Verification items for the finished model (mm, model axes). A direction names the side the tool comes from. Round coordinates to 2 decimals unless told otherwise and drop trailing zeros. Write each loop counter-clockwise with the first axis right and the second up, starting at its lowest first coordinate (ties: lowest second). Pieces come first, ordered by that corner, then holes. Notation, with made-up numbers: M 21.5,48 L 60.5,48 A11 ccw 60.5,64 Z; hole C 20,47.5 d3. An arc over 180 degrees is marked long. One line per question, with ' | ' between items.
Autodesk Inventor part; units mm, degrees
ref_plane "YZ Plane" through (0, 0, 0) normal (1, 0, 0) x (0, 1, 0)
ref_plane "XZ Plane" through (0, 0, 0) normal (0, 1, 0) x (-1, 0, 0)
ref_plane "XY Plane" through (0, 0, 0) normal (0, 0, 1) x (1, 0, 0)
sketch "Sketch1" plane through (0, 0, 0) normal (0, 1, 0) x (-1, 0, 0)
  line L0 (-2.45, -18) -> (2.45, -18)
  line L1 (2.45, -18) -> (2.45, 18)
  line L2 (2.45, 18) -> (-2.45, 18)
  line L3 (-2.45, 18) -> (-2.45, -18)
  line L4 (-2.45, -18) -> (2.45, 18) construction
  line L5 (2.45, -18) -> (-2.45, 18) construction
  point P0 (0, 0)
  dimension "d0" = 36
  dimension "d1" = 4.9
extrude "Extrusion1" add sketch "Sketch1" along normal blind 12
sketch "Sketch2" plane through (2.45, 0, 18) normal (1, 0, 0) x (0, 0, -1)
  circle A0 centre (26, 7) radius 2.5
  line L0 (36, 0) -> (36, 12)
  line L1 (0, 12) -> (36, 12)
  point P0 (18, 0)
  dimension "d4" = 5
  dimension "d5" = 10
  dimension "d18" = 5
fillet "Fillet1" radius 5 2 edges at (0, 12, -18) (0, 0, -18)
sketch "Sketch3" plane through (2.45, 0, 18) normal (1, 0, 0) x (0, 0, -1)
  line L0 (0, 0) -> (0, -15)
  arc A0 (36, 7) -> (31, 12) centre (31, 7) ccw
  line L1 (0, -15) -> (31, 0)
  line L2 (0, 0) -> (31, 0)
  point P0 (18, 0)
  dimension "d7" = 15
extrude "Extrusion2" cut sketch "Sketch2" against normal blind 10
extrude "Extrusion3" add sketch "Sketch3" against normal blind 5
sketch "Skizze4" plane through (2.45, 12, 18) normal (1, 0, 0) x (0, 0, -1)
  line L0 (8, -10) -> (3, -10)
  line L1 (3, -10) -> (3, -5)
  line L2 (3, -5) -> (8, -5)
  line L3 (8, -5) -> (8, -10)
  line L4 (0, 0) -> (31, 0)
  line L5 (0, -27) -> (0, 0)
  point P0 (18, -12)
  point P1 (3, -7.5)
  dimension "d12" = 5
  dimension "d13" = 5
  dimension "d14" = 5
  dimension "d15" = 3
extrude "Extrusion4" add sketch "Skizze4" along normal blind 5
sketch "Sketch5" plane through (-2.45, 5, -18) normal (-1, 0, 0) x (0, 0, 1)
  circle A0 centre (10, 2) radius 2.5
  arc A1 (0, 0) -> (5, -5) centre (5, 0) ccw
  line L0 (5, -5) -> (36, -5)
  line L1 (36, -5) -> (36, 7)
  line L2 (5, 7) -> (36, 7)
  arc A2 (5, 7) -> (0, 2) centre (5, 2) ccw
  line L3 (0, 0) -> (0, 2)
  line L4 (5, -5) -> (36, -20)
  line L5 (36, -20) -> (36, -5)
  line L6 (36, -5) -> (5, -5)
  line L7 (5, -5) -> (36, -20)
  line L8 (36, -20) -> (36, -5)
  line L9 (36, -5) -> (5, -5)
  line L10 (5, -5) -> (36, -20)
  line L11 (36, -20) -> (36, -5)
  line L12 (36, -5) -> (5, -5)
  point P0 (18, -5)
extrude "Extrusion5" add sketch "Sketch5" along normal blind 1.5
sketch "Sketch6" plane through (-3.95, 5, -18) normal (-1, 0, 0) x (0, 0, 1)
  line L0 (5, -5) -> (36, -20)
  line L1 (36, -20) -> (36, 7)
  line L2 (36, 7) -> (5, 7)
  arc A0 (5, 7) -> (0, 2) centre (5, 2) ccw
  line L3 (0, 2) -> (0, 0)
  arc A1 (0, 0) -> (5, -5) centre (5, 0) ccw
  circle A2 centre (10, 2) radius 2.5
  point P0 (18, -5)
extrude "Extrusion6" add sketch "Sketch6" along normal blind 0.1
sketch "Sketch7" plane through (2.45, 2, 10) normal (0, -1, 0) x (1, 0, 0)
  line L0 (0, 0) -> (0, 5)
  line L1 (0, 0) -> (5, 0)
  line L2 (5, 5) -> (5, 0)
  line L3 (0, 5) -> (5, 5)
  point P0 (-2.45, -10)
extrude "Extrusion7" add sketch "Sketch7" along normal blind 5
chamfer "Chamfer1" distance 5 angle 45 1 edges at (7.45, -3, 12.5)
sketch "Sketch8" plane through (-4.05, 5, -18) normal (-1, 0, 0) x (0, 0, 1)
  line L0 (36, -20) -> (36, 7)
  line L1 (36, 7) -> (5, 7)
  arc A0 (5, 7) -> (0, 2) centre (5, 2) ccw
  line L2 (0, 2) -> (0, 0)
  arc A1 (0, 0) -> (5, -5) centre (5, 0) ccw
  line L3 (5, -5) -> (36, -20)
  circle A2 centre (10, 2) radius 2.5
  point P0 (18, -5)
extrude "Extrusion8" add sketch "Sketch8" along normal blind 3.4
sketch "Sketch9" plane through (7.45, 12, 18) normal (1, 0, 0) x (0, 0, -1)
  line L0 (8, -10) -> (3, -10) construction
  line L1 (8, -5) -> (8, -10) construction
  line L2 (8, -5) -> (3, -5) construction
  line L3 (3, -5) -> (3, -10) construction
  line L4 (8, -10) -> (3, -10)
  line L5 (8, -5) -> (8, -10)
  line L6 (8, -5) -> (3, -5)
  line L7 (3, -5) -> (3, -10)
  point P0 (18, -12)
extrude "Extrusion9" add sketch "Sketch9" along normal blind 2.5
sketch "Sketch10" plane through (-7.45, 0, -13) normal (0, -0.9001593, -0.4355609) x (1, 0, 0)
  point P0 (7.45, 11.7021)
sketch "Sketch11" plane through (-7.45, 0, -13) normal (0, -0.9001593, -0.4355609) x (1, 0, 0)
  point P0 (7.45, 11.7021)
sketch "Sketch12" plane through (-7.45, 5, -18) normal (-1, 0, 0) x (0, 0, 1)
  line L0 (36, -20) -> (36, -25.5)
  line L1 (36, -25.5) -> (5, -10.5)
  line L2 (5, -10.5) -> (5, -5)
  arc A0 (0, 0) -> (5, -5) centre (5, 0) ccw
  line L3 (5, -5) -> (36, -20)
  point P0 (18, -5)
  dimension "d32" = 5.5
  dimension "d33" = 5.5
extrude "Extrusion10" add sketch "Sketch12" against normal blind 9.9
fillet "Fillet2" radius 5 1 edges at (-2.5, -5.5, -13)
fillet "Fillet3" [suppressed]
sketch "Sketch13" plane through (2.45, 5, -18) normal (1, 0, 0) x (0, 0, -1)
  line L0 (-36, 7) -> (-36, -25.5)
  line L1 (-36, 7) -> (-33, 7)
  line L2 (-33, 7) -> (-33, -17.5)
  line L3 (-33, -17.5) -> (-36, -17.5)
  line L4 (-36, -17.5) -> (-36, 7)
  point P0 (-18, -5)
  point P1 (-36, -17.5)
  dimension "d40" = 24.5
extrude "Extrusion11" cut sketch "Sketch13" against normal blind 10
chamfer "Chamfer2" distance 2 angle 45 1 edges at (-5.75, -12.5, 18)
properties part number "HoldingTri"
1. Thickness scan on line 1 (Z direction, x = -0.85, y = 7); line 2 (X direction, y = 9, z = -1.5); line 3 (Y direction, x = -5.7, z = -8). Record the ranges inside material, lowest first.
Results:
line 1: z = -18 to -10.5, -5.5 to 15 | line 2: x = -7.45 to 2.45 | line 3: y = -7.92 to 4.5, 9.5 to 12
2. Go/stop test with flat-tipped pins: P1, Ø1.5, axis at y = -5, z = -9, coming from the +X side; P2, Ø4, axis at x = 7, z = 13.5, coming from the +Y side; P3, Ø1.9, axis at x = -1, y = -1, coming from the -Z side. Record where each tip stops, or that it passes through.
Results:
P1: stops at x = 2.45 | P2: stops at y = 7 | P3: stops at z = -13
3. Section check C-C, the plane y = -5. Record the cut outline in (x, z), then the cut area to 3 significant figures.
Results:
outline: M -7.45,-12.25 L 2.45,-12.25 L 2.45,15 L -7.45,15 Z | area: 270 mm2
4. Section check A-A, the plane z = -8. Record the cut outline in (x, y), then the cut area to 3 significant figures.
Results:
outline: M -7.45,-7.92 L 2.45,-7.92 L 2.45,4.5 L -7.45,4.5 Z; M -7.45,9.5 L 2.45,9.5 L 2.45,12 L -7.45,12 Z | area: 148 mm2
5. Tool access check on faces 1 (the face through (-3, -1, -13)), 2 (the face through (5, 3, 10)), 3 (the face through (-1, 0, 15)). Record the directions out of +Z, -Z, +X, -X, +Y, -Y that give a thin tool (end or side, any length) a straight path to the whole face; none if there is none.
Results:
face 1: -Z, +X, -X, -Y | face 2: -Z, +X, +Y, -Y | face 3: +Z, +X, -X, +Y
6. Section check B-B, the plane x = -4.75. Record the cut outline in (y, z), then the cut area to 3 significant figures.
Results:
outline: M -20.5,18 L -6.87,-10.18 A5 ccw -2.36,-13 L 0,-13 A5 ccw 5,-18 L 7,-18 A5 ccw 12,-13 L 12,15 L -12.5,15 L -12.5,16 L -14.5,18 Z; hole C 7,-8 d5 | area: 727 mm2
7. Section check D-D, the plane z = -12.5. Record the cut outline in (x, y).
Results:
outline: M -7.45,-4.54 L 2.45,-4.54 L 2.45,12 L -7.45,12 Z
